Source: CAD feature listing. Evaluate the final solid. Frame: model axes, mm. A direction names the side the tool comes from. Give positions to 0.01 mm unless a question says otherwise; leave off trailing zeros. Write each loop counter-clockwise with the first axis right and the second up, starting at its lowest first coordinate (ties: lowest second). Pieces come first, ordered by that corner, then holes. Notation, with made-up numbers: M 42.5,43.5 L 49.5,43.5 A11 cw 49.5,55.5 Z; hole C 42,40.5 d2. An arc over 180 degrees is marked long. Return JSON: item names as keys, results as strings.
```python
from build123d import *

# Parameters (mm, degrees)
SKETCH2_R           = 2.38125
SKETCH2_R_2         = 1.8
SKETCH2_R_3         = 1.7
BOSS_EXTRUDE1_DEPTH = 6.35
FILLET1_R           = 5


with BuildPart() as part:
    # Sketch2 → Boss-Extrude1 (new body)
    with BuildSketch(Plane(origin=(0, 0, 0), x_dir=(1, 0, 0), z_dir=(0, 1, 0))):
        Polygon((-85.5, -90), (100, -90), (100, 90), (-85.5, 90), (-85.5, 30.004081815), (-100, 30.004081815), (-100, -30.004081815), (-85.5, -30.004081815), align=None)
        with Locations(Location((-81, -64, 0), (0, 0, 270))):
            Circle(SKETCH2_R, mode=Mode.SUBTRACT)
        with Locations(Location((-81, -57, 0), (0, 0, 270))):
            Circle(SKETCH2_R, mode=Mode.SUBTRACT)
        with Locations(Location((-9.5, -85, 0), (0, 0, 270))):
            Circle(SKETCH2_R_2, mode=Mode.SUBTRACT)
        with Locations(Location((-95, -9.5, 0), (0, 0, 270))):
            Circle(SKETCH2_R_2, mode=Mode.SUBTRACT)
        with Locations(Location((-86, -8, 0), (0, 0, 270))):
            Circle(SKETCH2_R_3, mode=Mode.SUBTRACT)
        with Locations(Location((9.5, -85, 0), (0, 0, 270))):
            Circle(SKETCH2_R_2, mode=Mode.SUBTRACT)
        with Locations(Location((86, -8, 0), (0, 0, 270))):
            Circle(SKETCH2_R_3, mode=Mode.SUBTRACT)
        with Locations(Location((95, -9.5, 0), (0, 0, 270))):
            Circle(SKETCH2_R_2, mode=Mode.SUBTRACT)
        with Locations(Location((-95, 9.5, 0), (0, 0, 270))):
            Circle(SKETCH2_R_2, mode=Mode.SUBTRACT)
        with Locations(Location((-86, 8, 0), (0, 0, 270))):
            Circle(SKETCH2_R_3, mode=Mode.SUBTRACT)
        with Locations(Location((-81, 57, 0), (0, 0, 270))):
            Circle(SKETCH2_R, mode=Mode.SUBTRACT)
        with Locations(Location((-81, 64, 0), (0, 0, 270))):
            Circle(SKETCH2_R, mode=Mode.SUBTRACT)
        with Locations(Location((-9.5, 85, 0), (0, 0, 270))):
            Circle(SKETCH2_R_2, mode=Mode.SUBTRACT)
        with Locations(Location((86, 8, 0), (0, 0, 270))):
            Circle(SKETCH2_R_3, mode=Mode.SUBTRACT)
        with Locations(Location((95, 9.5, 0), (0, 0, 270))):
            Circle(SKETCH2_R_2, mode=Mode.SUBTRACT)
        with Locations(Location((9.5, 85, 0), (0, 0, 270))):
            Circle(SKETCH2_R_2, mode=Mode.SUBTRACT)
    extrude(amount=BOSS_EXTRUDE1_DEPTH)

    # Fillet1
    fillet1_edges = [part.edges().sort_by_distance(p)[0] for p in [
        (-100, 3.175, 30.004081815),
        (-100, 3.175, -30.004081815),
        (-85.5, 3.175, -90),
        (100, 3.175, -90),
        (100, 3.175, 90),
        (-85.5, 3.175, 90),
    ]]
    fillet(fillet1_edges, radius=FILLET1_R)


solid = part.part
```
1) Contact query for a flat-ended pin moving along its axis: pin 1 Ø4 at (x, z) = (-81, 64) entering from -Y. Output: stop coordinate, or through.
Numbers:
{"pin 1": "passes through"}
2) Cut plane A-A, the plane y = 2.5. Give the number of separate pieces and of enclosed holes in the cut face, then the cut area to 3 significant figures.
Numbers:
{"separate pieces": "1", "enclosed holes": "16", "area": "34,000 mm²"}
3) Cut plane B-B, the plane z = -70.5. Return the cut outline in (x, y), then the cut area to 3 significant figures.
Numbers:
{"outline": "M -85.5,0 L 100,0 L 100,6.35 L -85.5,6.35 Z", "area": "1,180 mm²"}
4) Line query: line 1 (Z direction, x = -95, y = 5); line 2 (X direction, y = 2.5, z = 85); line 3 (Z direction, x = 95, y = 3.25). Output: solid intervals per line, ascending. Write a range as [from, to].
Numbers:
{"line 1": "z = [-30, -11.3], [-7.7, 7.7], [11.3, 30]", "line 2": "x = [-85.5, -11.3], [-7.7, 7.7], [11.3, 100]", "line 3": "z = [-90, -11.3], [-7.7, 7.7], [11.3, 90]"}
5) Draft query along Z for faces 1 (the face through (-80.9, 3.13, 54.62)), 2 (the face through (-85.5, 3, -58)), 3 (the face through (-90, 3, 30.004)), 4 (the face through (-98.574, 3.219, -28.501)). Return one class per face: released by +Z, released by -Z, zero draft, split by the parting line, or undercut.
Numbers:
{"face 1": "undercut", "face 2": "zero draft", "face 3": "released by +Z", "face 4": "released by -Z"}
6) Set-up query: faces 5 (the face through (-85.5, 3, 57)), 6 (the face through (-83.325, 3.131, 63.484)). Return all of +Z, -Z, +X, -X, +Y, -Y with unobstructed straight access to the full face (end or side cutting, diameter ignored); none if empty.
Numbers:
{"face 5": "+Z, -X, +Y, -Y", "face 6": "+Y, -Y"}
